Could you check a few things on this model? Use its own coordinates, in mm. Face numbers are marked on the shaded views. Coordinates: 2 decimals unless noted, no trailing zeros. Order: outer loops, then holes, each group sorted by start corner. A loop starts at its lowest first (then second) coordinate and runs counter-clockwise, first axis right, second up. Notation, with made-up numbers: M 4.25,-35 L 41.25,-35 A23 ccw 41.25,1 Z; hole C 80,-2 d11. An arc over 180 degrees is marked long. Write item = value, one per line. Start each with the question number.
from build123d import *

# Parameters (mm, degrees)
SKETCH1_W                  = 65.44
SKETCH1_H                  = 122
BOSS_EXTRUDE1_DEPTH        = 20
M5X0_8_TAPPED_HOLE1_D      = 4.2
M5X0_8_TAPPED_HOLE1_DEPTH  = 20
M8X1_25_TAPPED_HOLE1_D     = 6.8
M8X1_25_TAPPED_HOLE1_DEPTH = 20


with BuildPart() as part:
    # Sketch1 → Boss-Extrude1 (new body)
    with BuildSketch(Plane.XY):
        Rectangle(SKETCH1_W, SKETCH1_H)
    extrude(amount=BOSS_EXTRUDE1_DEPTH)

    # M5x0.8 Tapped Hole1
    with Locations(Plane.XY.offset(20)):
        with Locations((0, 20), (-17.320508076, 10), (-17.320508076, -10), (0, -20), (17.320508076, -10), (17.320508076, 10)):
            Hole(M5X0_8_TAPPED_HOLE1_D / 2, depth=M5X0_8_TAPPED_HOLE1_DEPTH)

    # M8x1.25 Tapped Hole1
    with Locations(Plane.XY.offset(20)):
        with Locations((-15.37, 53), (15.37, 53), (15.37, -53), (-15.37, -53)):
            Hole(M8X1_25_TAPPED_HOLE1_D / 2, depth=M8X1_25_TAPPED_HOLE1_DEPTH)


solid = part.part
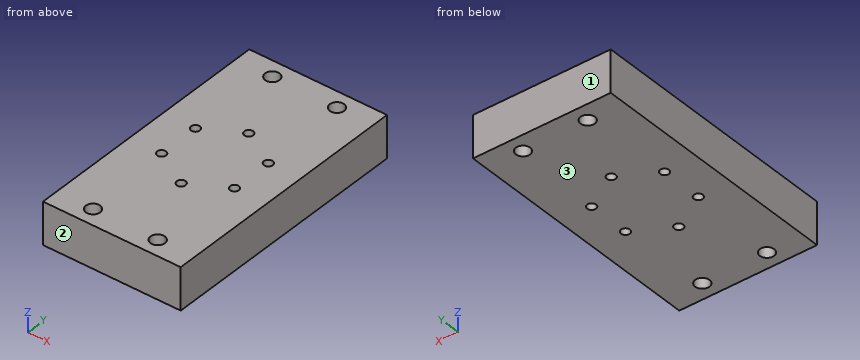
(1) Imagine slicing it at B-B on z = 15. Give the number of separate pieces and of enclosed holes in the cut face, plus the area to 3 significant figures.
(2) Thinking about a two-plate mould opening in Y: for the marked faces 1, 2 and 3, which applies, released by +Y, released by -Y, zero draft, split by the parting line, or undercut?
(3) Please list where these lines run through material, in increasing order: probe 1 along X at (y, z) = (-9.5, 1); probe 2 along X at (y, z) = (-52, 14.25); probe 3 along Y at (x, z) = (1, 2). Write a range as from..to.
(4) Imagine slicing it at A-A on y = 20. List the corners of the cut face in (x, z) for me.
Response:
q1.separate_pieces = 1
q1.enclosed_holes = 10
q1.area = 7,760 mm2
q2.face_1 = released by +Y
q2.face_2 = released by -Y
q2.face_3 = zero draft
q3.probe_1 = -32.72..-19.36, -15.28..15.28, 19.36..32.72
q3.probe_2 = -32.72..-18.62, -12.12..12.12, 18.62..32.72
q3.probe_3 = -61..-21.85, -18.15..18.15, 21.85..61
q4.outline = M -32.72,0 L -2.1,0 L -2.1,20 L -32.72,20 Z; M 2.1,0 L 32.72,0 L 32.72,20 L 2.1,20 Z
